Geometry check sheet. Reference: the model listing, model coordinates, mm. A direction names the side the tool comes from. Round coordinates to 2 decimals unless told otherwise and drop trailing zeros. Order: outer loops, then holes, each group sorted by start corner. A loop starts at its lowest first (then second) coordinate and runs counter-clockwise, first axis right, second up. Notation, with made-up numbers: (85, 31.5) - (101, 31.5) arc R22 ccw to (101, 59.5) - close; hole circle Ø1 at (55, 47.25). An arc over 180 degrees is marked (long way). One line per question, with ' | ' between items. Start each with the question number.
Q1. Tool access check on faces 1 (the face through (0.05, 30, 5)), 2 (the face through (8.74, -2.17, 0.41)), 3 (the face through (0.85, 27.6, 5.6)). Record the directions out of +Z, -Z, +X, -X, +Y, -Y that give a thin tool (end or side, any length) a straight path to the whole face; none if there is none.
Q2. Material ranges on line 1 along Y through (x, z) = (8.6, 0.2) (3 decimals); line 2 along X through (y, z) = (13, 0.5); line 3 along Z through (x, y) = (0.7, 28.75), recorded low to high.
Q3. Mould release check, pull along Y, two halves, no side actions. Record for faces 4 (the face through (16.476, -12.711, 0.394)), 5 (the face through (16, 14, 0)), 6 (the face through (8.456, 29.195, 0.406)): +Y half, -Y half, draft (parallel to the pull), parting line (faces both ways), or undercut.
Q4. Sectioned sample at A-A, the plane y = 10. Enter the section's corners in (x, z), then the cut area to 3 significant figures.
Q5. Sectioned sample at B-B, the plane z = 3.5. Enter the section's corners in (x, y).
Q6. Gauge pin test, flat ends, axial feed: P1, Ø2.5, axis at y = 30.5, z = 7.5, coming from the +X side; P2, Ø0.9, axis at y = 23.5, z = 0.5, coming from the -X side; P3, Ø3, axis at x = 15, y = 4.5, coming from the +Z side. Record the tip position at first contact, or that the pin passes through.
Q7. Sectioned sample at C-C, the plane x = 8.6. Enter the section's corners in (y, z) (3 decimals).
```python
from build123d import *

# Parameters (mm, degrees)
BOSS_EXTRUDE1_START             = -0.8
BOSS_EXTRUDE1_DEPTH             = 1
BOSS_EXTRUDE1_2_OUTLINE_W       = 0.8
BOSS_EXTRUDE1_2_OUTLINE_H       = 9.5
BOSS_EXTRUDE1_2_DEPTH           = 9.2
BOSS_EXTRUDE1_START_2           = 0.85
BOSS_EXTRUDE1_3_OUTLINE_W       = 40.5
BOSS_EXTRUDE1_3_OUTLINE_H       = 0.2
BOSS_EXTRUDE1_3_DEPTH           = 15.5
BOSS_EXTRUDE1_4_OUTLINE_R       = 1
BOSS_EXTRUDE1_4_OUTLINE_W       = 22
BOSS_EXTRUDE1_4_OUTLINE_H       = 0.2
BOSS_EXTRUDE1_4_DEPTH           = 17.2
BOSS_EXTRUDE1_START_3           = 17.112671
BOSS_EXTRUDE1_5_OUTLINE_W       = 9.5
BOSS_EXTRUDE1_5_OUTLINE_H       = 0.2
BOSS_EXTRUDE1_5_DEPTH           = 0.037329
BOSS_EXTRUDE1_START_4           = 0.05
BOSS_EXTRUDE1_6_OUTLINE_W       = 9.5
BOSS_EXTRUDE1_6_OUTLINE_H       = 0.2
BOSS_EXTRUDE1_6_DEPTH           = 0.032671
BOSS_EXTRUDE1_START_5           = 24
BOSS_EXTRUDE1_7_DEPTH           = 9.5
BOSS_EXTRUDE1_8_DEPTH           = 9.5
SKETCH2_W                       = 17.2
SKETCH2_H                       = 35.475
BOSS_EXTRUDE2_DEPTH             = 0.8
FILLET1_R                       = 2.54
F_5_32_0_15625_DIAMETER_HOLE1_D = 3.96875
CUT_EXTRUDE1_DEPTH              = 45.952530518


with BuildPart() as part:
    # Boss-Extrude1: read off the stored shape, not the designer's step
    # Boss-Extrude1 outline → Boss-Extrude1 (new body)
    with BuildSketch(Plane.XY.offset(0.8).offset(BOSS_EXTRUDE1_START)):
        with BuildLine():
            Line((0.05, 24), (1.06, 24))
            Line((1.06, 24), (1.06, 23.99))
            Line((1.06, 23.99), (0.85, 23.99))
            Line((0.85, 23.99), (0.85, 22))
            Line((0.85, 22), (0, 22))
            Line((0, 22), (0, 2))
            ThreePointArc((0, 2), (0.585786438, 0.585786438), (2, 0))
            Line((2, 0), (15.2, 0))
            ThreePointArc((15.2, 0), (16.614213562, 0.585786438), (17.2, 2))
            Line((17.2, 2), (17.2, 22))
            Line((17.2, 22), (16.35, 22))
            Line((16.35, 22), (16.35, 23.99))
            Line((16.35, 23.99), (16.14, 23.99))
            Line((16.14, 23.99), (16.14, 24))
            Line((16.14, 24), (17.15, 24))
            Line((17.15, 24), (17.15, 33.5))
            Line((17.15, 33.5), (16.14, 33.5))
            Line((16.14, 33.5), (16.14, 33.51))
            Line((16.14, 33.51), (16.35, 33.51))
            Line((16.35, 33.51), (16.35, 38.5))
            ThreePointArc((16.35, 38.5), (15.764213562, 39.914213562), (14.35, 40.5))
            Line((14.35, 40.5), (2.85, 40.5))
            ThreePointArc((2.85, 40.5), (1.435786438, 39.914213562), (0.85, 38.5))
            Line((0.85, 38.5), (0.85, 33.51))
            Line((0.85, 33.51), (1.06, 33.51))
            Line((1.06, 33.51), (1.06, 33.5))
            Line((1.06, 33.5), (0.05, 33.5))
            Line((0.05, 33.5), (0.05, 24))
        make_face()
    extrude(amount=BOSS_EXTRUDE1_DEPTH)

    # Boss-Extrude1 2 outline → Boss-Extrude1 2 (add)
    with BuildSketch(Plane.XY.offset(0.8)):
        with Locations((0.45, 28.75)):
            Rectangle(BOSS_EXTRUDE1_2_OUTLINE_W, BOSS_EXTRUDE1_2_OUTLINE_H)
        with Locations((16.75, 28.75)):
            Rectangle(BOSS_EXTRUDE1_2_OUTLINE_W, BOSS_EXTRUDE1_2_OUTLINE_H)
    extrude(amount=BOSS_EXTRUDE1_2_DEPTH)

    # Boss-Extrude1 3 outline → Boss-Extrude1 3 (cut)
    with BuildSketch(Plane.YZ.offset(BOSS_EXTRUDE1_START_2)):
        with Locations((20.25, 0.9)):
            Rectangle(BOSS_EXTRUDE1_3_OUTLINE_W, BOSS_EXTRUDE1_3_OUTLINE_H)
    extrude(amount=BOSS_EXTRUDE1_3_DEPTH, mode=Mode.SUBTRACT)

    # Boss-Extrude1 4 outline → Boss-Extrude1 4 (cut)
    with BuildSketch(Plane.YZ):
        with Locations((28.75, 5.25)):
            Circle(BOSS_EXTRUDE1_4_OUTLINE_R)
        with BuildLine():
            ThreePointArc((28.75, 10), (32.108757211, 8.608757211), (33.5, 5.25))
            Line((33.5, 5.25), (33.5, 10))
            Line((33.5, 10), (28.75, 10))
        make_face()
        with BuildLine():
            ThreePointArc((24, 5.25), (25.391242789, 8.608757211), (28.75, 10))
            Line((28.75, 10), (24, 10))
            Line((24, 10), (24, 5.25))
        make_face()
        with Locations((11, 0.9)):
            Rectangle(BOSS_EXTRUDE1_4_OUTLINE_W, BOSS_EXTRUDE1_4_OUTLINE_H)
    extrude(amount=BOSS_EXTRUDE1_4_DEPTH, mode=Mode.SUBTRACT)

    # Boss-Extrude1 5 outline → Boss-Extrude1 5 (cut)
    with BuildSketch(Plane.YZ.offset(BOSS_EXTRUDE1_START_3)):
        with Locations((28.75, 0.9)):
            Rectangle(BOSS_EXTRUDE1_5_OUTLINE_W, BOSS_EXTRUDE1_5_OUTLINE_H)
    extrude(amount=BOSS_EXTRUDE1_5_DEPTH, mode=Mode.SUBTRACT)

    # Boss-Extrude1 6 outline → Boss-Extrude1 6 (cut)
    with BuildSketch(Plane.YZ.offset(BOSS_EXTRUDE1_START_4)):
        with Locations((28.75, 0.9)):
            Rectangle(BOSS_EXTRUDE1_6_OUTLINE_W, BOSS_EXTRUDE1_6_OUTLINE_H)
    extrude(amount=BOSS_EXTRUDE1_6_DEPTH, mode=Mode.SUBTRACT)

    # Boss-Extrude1 7 outline → Boss-Extrude1 7 (cut)
    with BuildSketch(Plane(origin=(0, 0, 0), x_dir=(1, 0, 0), z_dir=(0, 1, 0)).offset(BOSS_EXTRUDE1_START_5)):
        with BuildLine():
            Line((0.05, -0.8), (0.070204103, -0.8))
            ThreePointArc((0.070204103, -0.8), (0.417544468, -0.225403331), (1.05, 0))
            Line((1.05, 0), (0.05, 0))
            Line((0.05, 0), (0.05, -0.8))
        make_face()
        with BuildLine():
            ThreePointArc((16.15, 0), (16.782455532, -0.225403331), (17.129795897, -0.8))
            Line((17.129795897, -0.8), (17.15, -0.8))
            Line((17.15, -0.8), (17.15, 0))
            Line((17.15, 0), (16.15, 0))
        make_face()
    extrude(amount=BOSS_EXTRUDE1_7_DEPTH, mode=Mode.SUBTRACT)

    # Boss-Extrude1 8 outline → Boss-Extrude1 8 (add)
    with BuildSketch(Plane(origin=(0, 0, 0), x_dir=(1, 0, 0), z_dir=(0, 1, 0)).offset(BOSS_EXTRUDE1_START_5)):
        with BuildLine():
            Line((0.85, -0.8), (0.85, -1))
            ThreePointArc((0.85, -1), (0.908578644, -0.858578644), (1.05, -0.8))
            Line((1.05, -0.8), (0.85, -0.8))
        make_face()
        with BuildLine():
            Line((16.35, -0.8), (16.15, -0.8))
            ThreePointArc((16.15, -0.8), (16.291421356, -0.858578644), (16.35, -1))
            Line((16.35, -1), (16.35, -0.8))
        make_face()
        with BuildLine():
            Line((0.082671, -1), (0.082671, -0.8))
            Line((0.082671, -0.8), (0.070204103, -0.8))
            ThreePointArc((0.070204103, -0.8), (0.055063847, -0.899491038), (0.05, -1))
            Line((0.05, -1), (0.082671, -1))
        make_face()
        with BuildLine():
            Line((17.129795897, -0.8), (17.112671, -0.8))
            Line((17.112671, -0.8), (17.112671, -1))
            Line((17.112671, -1), (17.15, -1))
            ThreePointArc((17.15, -1), (17.144936153, -0.899491038), (17.129795897, -0.8))
        make_face()
    extrude(amount=BOSS_EXTRUDE1_8_DEPTH)

    # Sketch2 → Boss-Extrude2 (add)
    with BuildSketch(Plane.XY.offset(0.8)):
        with Locations((8.6, 4.2625)):
            Rectangle(SKETCH2_W, SKETCH2_H)
    extrude(amount=-BOSS_EXTRUDE2_DEPTH)

    # Fillet1
    fillet1_edges = [part.edges().sort_by_distance(p)[0] for p in [
        (0, -13.475, 0.4),
        (17.2, -13.475, 0.4),
    ]]
    fillet(fillet1_edges, radius=FILLET1_R)

    # 5/32 (0.15625) Diameter Hole1 (through all)
    with Locations(Plane.XY.offset(0.8)):
        with Locations((8.6, -9.5126), (8.6, 36.5122)):
            Hole(F_5_32_0_15625_DIAMETER_HOLE1_D / 2)

    # Sketch5 → Cut-Extrude1 (cut, through all)
    with BuildSketch(Plane.XY.offset(0.8)):
        with BuildLine():
            Line((2.0468, 4.3812), (2.0468, 22.6438))
            ThreePointArc((2.0468, 22.6438), (8.6, 29.197), (15.1532, 22.6438))
            Line((15.1532, 22.6438), (15.1532, 4.3812))
            ThreePointArc((15.1532, 4.3812), (8.6, -2.172), (2.0468, 4.3812))
        make_face()
    extrude(amount=-CUT_EXTRUDE1_DEPTH, mode=Mode.SUBTRACT)


solid = part.part
```
Determined:
1) face 1: +Z, -Z, -X, +Y, -Y | face 2: +Z, -Z | face 3: +Z, +Y, -Y
2) line 1: y = -13.475 to -11.497, -7.528 to -2.172, 29.197 to 34.528, 38.497 to 40.5 | line 2: x = 0 to 2.05, 15.15 to 17.2 | line 3: z = 0.06 to 4.25, 6.25 to 10
3) face 4: -Y half | face 5: draft | face 6: undercut
4) outline: (0, 0) - (2.05, 0) - (2.05, 0.8) - (0, 0.8) - close; (15.15, 0) - (17.2, 0) - (17.2, 0.8) - (15.15, 0.8) - close | area: 3.27 mm2
5) outline: (0.05, 24) - (0.85, 24) - (0.85, 33.5) - (0.05, 33.5) - close; (16.35, 24) - (17.15, 24) - (17.15, 33.5) - (16.35, 33.5) - close
6) P1: stops at x = 17.15 | P2: stops at x = 0.85 | P3: stops at z = 0.8
7) outline: (-13.475, 0) - (-11.497, 0) - (-11.497, 0.8) - (-13.475, 0.8) - close; (-7.528, 0) - (-2.172, 0) - (-2.172, 0.8) - (-7.528, 0.8) - close; (29.197, 0) - (34.528, 0) - (34.528, 0.8) - (29.197, 0.8) - close; (38.497, 0) - (40.5, 0) - (40.5, 0.8) - (38.497, 0.8) - close
